Build history of the part. All positions in model axes, mm. Round coordinates to 2 decimals unless told otherwise and drop trailing zeros. Order: outer loops, then holes, each group sorted by start corner. A loop starts at its lowest first (then second) coordinate and runs counter-clockwise, first axis right, second up. Notation, with made-up numbers: (-36.5, 62.25) - (-15.5, 62.25) arc R20 ccw to (-15.5, 78.25) - close; hole circle Ø1 at (-25, -5.75). An arc over 180 degrees is marked (long way). One line per question, with ' | ' between items. Start each with the question number.
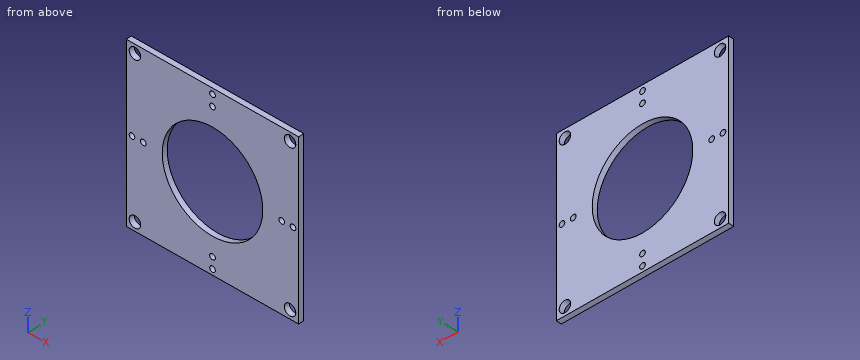
from build123d import *

# Parameters (mm, degrees)
SKETCH1_W           = 152.4
SKETCH1_H           = 152.4
SKETCH1_R           = 44.45
SKETCH1_R_2         = 2.5
SKETCH1_R_3         = 5.08
BOSS_EXTRUDE1_DEPTH = 4.7498


with BuildPart() as part:
    # Sketch1 → Boss-Extrude1 (new body)
    with BuildSketch(Plane(origin=(0, 0, 0), x_dir=(1, 0, 0), z_dir=(0, 1, 0))):
        Rectangle(SKETCH1_W, SKETCH1_H)
        with Locations(Location((0, 0, 0), (0, 0, 270))):
            Circle(SKETCH1_R, mode=Mode.SUBTRACT)
        with Locations(Location((0, -71.2, 0), (0, 0, 270))):
            Circle(SKETCH1_R_2, mode=Mode.SUBTRACT)
        with Locations(Location((0, -61.2, 0), (0, 0, 270))):
            Circle(SKETCH1_R_2, mode=Mode.SUBTRACT)
        with Locations(Location((-61.2, 0, 0), (0, 0, 270))):
            Circle(SKETCH1_R_2, mode=Mode.SUBTRACT)
        with Locations(Location((-71.2, 0, 0), (0, 0, 270))):
            Circle(SKETCH1_R_2, mode=Mode.SUBTRACT)
        with Locations(Location((0, 61.2, 0), (0, 0, 270))):
            Circle(SKETCH1_R_2, mode=Mode.SUBTRACT)
        with Locations(Location((0, 71.2, 0), (0, 0, 270))):
            Circle(SKETCH1_R_2, mode=Mode.SUBTRACT)
        with Locations(Location((61.2, 0, 0), (0, 0, 270))):
            Circle(SKETCH1_R_2, mode=Mode.SUBTRACT)
        with Locations(Location((71.2, 0, 0), (0, 0, 270))):
            Circle(SKETCH1_R_2, mode=Mode.SUBTRACT)
        with Locations(Location((-68.58, -68.58, 0), (0, 0, 270))):
            Circle(SKETCH1_R_3, mode=Mode.SUBTRACT)
        with Locations(Location((-68.58, 68.58, 0), (0, 0, 270))):
            Circle(SKETCH1_R_3, mode=Mode.SUBTRACT)
        with Locations(Location((68.58, 68.58, 0), (0, 0, 270))):
            Circle(SKETCH1_R_3, mode=Mode.SUBTRACT)
        with Locations(Location((68.58, -68.58, 0), (0, 0, 270))):
            Circle(SKETCH1_R_3, mode=Mode.SUBTRACT)
    extrude(amount=BOSS_EXTRUDE1_DEPTH)


solid = part.part
Item 1: Slice it at B-B (y = 2.5). Count the separate pieces of the cut face and the enclosed holes in it, plus the area to 3 significant figures.
Item 2: Wall check: line 1 along X through (y, z) = (1.7, -68.58); line 2 along Z through (x, y) = (70.5, 4.5); line 3 along X through (y, z) = (1.65, 0). Give the ranges that are in metal, low to high. Write a range as [from, to].
Item 3: Slice it at A-A (z = 61.2). Write the cut outline in (x, y).
Item 4: Slice it at C-C (x = 0). Write the cut outline in (y, z).
Item 5: Slice it at D-D (z = 0). Write the cut outline in (x, y), plus the area to 3 significant figures.
A:
1) separate pieces: 1 | enclosed holes: 13 | area: 16,500 mm^2
2) line 1: [-76.2, -73.66], [-63.5, 63.5], [73.66, 76.2] | line 2: [-76.2, -73.28], [-63.88, -2.4], [2.4, 63.88], [73.28, 76.2] | line 3: [-76.2, -73.7], [-68.7, -63.7], [-58.7, -44.45], [44.45, 58.7], [63.7, 68.7], [73.7, 76.2]
3) outline: (-76.2, 0) - (-2.5, 0) - (-2.5, 4.75) - (-76.2, 4.75) - close; (2.5, 0) - (76.2, 0) - (76.2, 4.75) - (2.5, 4.75) - close
4) outline: (0, -76.2) - (4.75, -76.2) - (4.75, -73.7) - (0, -73.7) - close; (0, -68.7) - (4.75, -68.7) - (4.75, -63.7) - (0, -63.7) - close; (0, -58.7) - (4.75, -58.7) - (4.75, -44.45) - (0, -44.45) - close; (0, 44.45) - (4.75, 44.45) - (4.75, 58.7) - (0, 58.7) - close; (0, 63.7) - (4.75, 63.7) - (4.75, 68.7) - (0, 68.7) - close; (0, 73.7) - (4.75, 73.7) - (4.75, 76.2) - (0, 76.2) - close
5) outline: (-76.2, 0) - (-73.7, 0) - (-73.7, 4.75) - (-76.2, 4.75) - close; (-68.7, 0) - (-63.7, 0) - (-63.7, 4.75) - (-68.7, 4.75) - close; (-58.7, 0) - (-44.45, 0) - (-44.45, 4.75) - (-58.7, 4.75) - close; (44.45, 0) - (58.7, 0) - (58.7, 4.75) - (44.45, 4.75) - close; (63.7, 0) - (68.7, 0) - (68.7, 4.75) - (63.7, 4.75) - close; (73.7, 0) - (76.2, 0) - (76.2, 4.75) - (73.7, 4.75) - close | area: 207 mm^2
